Input: dimensioned drawing with shaded views. Units: mm. Origin: part minimum x, y, z. A direction names the side the tool comes from. Round coordinates to 2 decimals unless told otherwise and drop trailing zeros. Loops run counter-clockwise (first coordinate to the right, second up) from the corner with the lowest first, then second, coordinate; pieces in that order, holes last. Notation, with made-up numbers: M 35.5,70.25 L 82.5,70.25 A36 ccw 82.5,108.25 Z; hole C 5.5,-13 d2. An arc over 180 degrees is marked long. Answer as a JSON object with one key per item and string values.
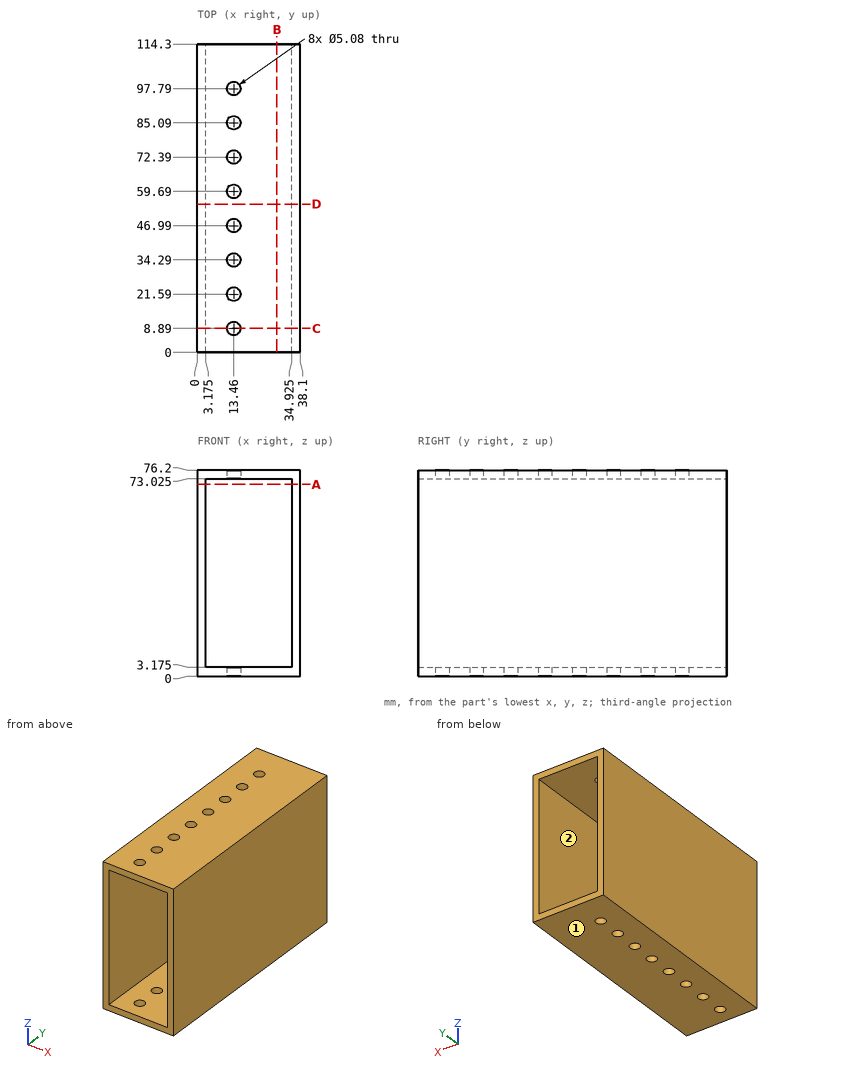
Item 1: Section B-B on x = 29.5. Return the cut outline in (y, z) (3 decimals), then the cut area to 3 significant figures.
Answer sheet:
{"outline": "M 0,0 L 114.3,0 L 114.3,3.175 L 0,3.175 Z; M 0,73.025 L 114.3,73.025 L 114.3,76.2 L 0,76.2 Z", "area": "726 mm²"}
Item 2: Access query for the marked faces 1 and 2. Directions: +Z, -Z, +X, -X, +Y, -Y. A direction counts if a zero-diameter tool reaches every point of the face in a straight line with its end or side. Return the directions, or none.
Answer sheet:
{"face 1": "-Z, +X, -X, +Y, -Y", "face 2": "+Y, -Y"}
Item 3: Contact query for a flat-ended pin moving along its axis: pin 1 Ø3 at (x, y) = (13.46, 85.09) entering from +Z. Output: stop coordinate, or through.
Answer sheet:
{"pin 1": "passes through"}
Item 4: Section C-C on y = 8.89. Return the cut outline in (x, z) (3 decimals), then the cut area to 3 significant figures.
Answer sheet:
{"outline": "M 0,0 L 10.92,0 L 10.92,3.175 L 3.175,3.175 L 3.175,73.025 L 10.92,73.025 L 10.92,76.2 L 0,76.2 Z; M 16,0 L 38.1,0 L 38.1,76.2 L 16,76.2 L 16,73.025 L 34.925,73.025 L 34.925,3.175 L 16,3.175 Z", "area": "653 mm²"}
Item 5: Section A-A on z = 71. Return the cut outline in (x, y) (3 decimals).
Answer sheet:
{"outline": "M 0,0 L 3.175,0 L 3.175,114.3 L 0,114.3 Z; M 34.925,0 L 38.1,0 L 38.1,114.3 L 34.925,114.3 Z"}
Item 6: Section D-D on y = 55. Return the cut outline in (x, z) (3 decimals), then the cut area to 3 significant figures.
Answer sheet:
{"outline": "M 0,0 L 38.1,0 L 38.1,76.2 L 0,76.2 Z; hole M 3.175,3.175 L 34.925,3.175 L 34.925,73.025 L 3.175,73.025 Z", "area": "685 mm²"}
Item 7: Line query: probe 1 along Z at (x, y) = (27, 89.5) (3 decimals); probe 2 along X at (y, z) = (88, 40) (3 decimals); probe 3 along X at (y, z) = (85, 1). Output: solid intervals per line, ascending. Write a range as from..to.
Answer sheet:
{"probe 1": "z = 0..3.175, 73.025..76.2", "probe 2": "x = 0..3.175, 34.925..38.1", "probe 3": "x = 0..10.92, 16..38.1"}
